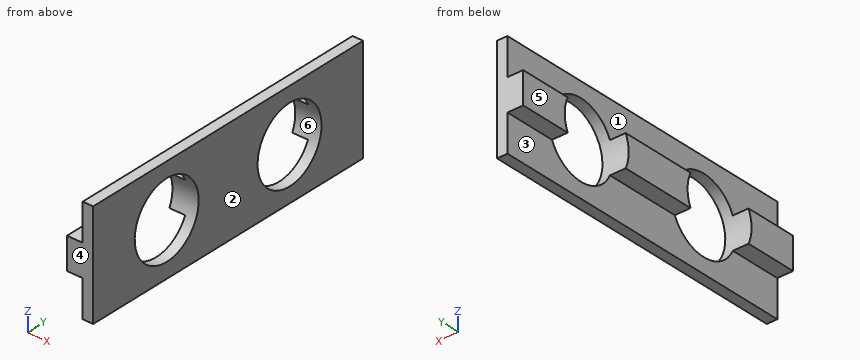
from build123d import *

# Parameters (mm, degrees)
BOSS_EXTRUDE1_DEPTH = 30
SKETCH2_R           = 3.556
CUT_EXTRUDE1_DEPTH  = 30


with BuildPart() as part:
    # Sketch1 → Boss-Extrude1 (new body)
    with BuildSketch(Plane(origin=(0, 0, 0), x_dir=(1, 0, 0), z_dir=(0, 1, 0))):
        Polygon((-1.62605042, 3), (-1.62605042, 6.5), (-0.62605042, 6.5), (-0.62605042, -3.5), (-1.62605042, -3.5), (-1.62605042, 0), (-3.12605042, 0), (-3.12605042, 3), align=None)
    extrude(amount=BOSS_EXTRUDE1_DEPTH)

    # Sketch2 → Cut-Extrude1 (cut)
    with BuildSketch(Plane.ZY.offset(3.12605042)):
        with Locations((-1.5, 21.829992104)):
            Circle(SKETCH2_R)
        with Locations((-1.5, 8.170007896)):
            Circle(SKETCH2_R)
    extrude(amount=-CUT_EXTRUDE1_DEPTH, mode=Mode.SUBTRACT)


solid = part.part
Could you check a few things on this model? Use its own coordinates, in mm. Face numbers are marked on the shaded views. A direction names the side the tool comes from. Coordinates: 2 decimals unless noted, no trailing zeros. Write each loop counter-clockwise with the first axis right and the second up, starting at its lowest first coordinate (ties: lowest second). Pieces come first, ordered by that corner, then holes. Notation, with made-up numbers: (60.5, -23.5) - (117.5, -23.5) arc R33 cw to (117.5, 11.5) - close; hole circle Ø4 at (37, 68). An arc over 180 degrees is marked (long way). Put each result on its own line as item: value. Start each with the question number.
Q1. I want a section at B-B on y = 20. Write out the boundary of the cut face in (x, z).
Q2. Thinking about a two-plate mould opening in Y: for the marked faces 4, 5 and 6, which applies, pulls with the +Y half, pulls with the -Y half, needs draft (parallel to the pull), parting line crosses it, or undercut?
Q3. Please list where these lines run through material, in increasing order: L1, parallel to Y at x = -2.5, z = -1.5; L2, parallel to Y at x = -1.45, z = 1.5; L3, parallel to Z at x = -1.4, y = 8.
Q4. Which directions (+Z, -Z, +X, -X, +Y, -Y) give clear straight access to the entire face, cutting with the end or side of a thin tool? Please do the marked faces 1, 2 and 3.
Q5. I want a section at C-C on z = 1.75. Write out the boundary of the cut face in (x, y).
Q6. I'm going to push flat-ended pins straight in: P1, Ø6, axis at y = 22, z = -0.5, coming from the -X side; P2, Ø5.5, axis at y = 21.83, z = -1.5, coming from the +X side. Where does each tip first touch, or does it pass through?
Q7. I want a section at A-A on x = -2.15. Write out the boundary of the cut face in (y, z).
Checks:
1. outline: (-1.63, -6.5) - (-0.63, -6.5) - (-0.63, -4.55) - (-1.63, -4.55) - close; (-1.63, 1.55) - (-0.63, 1.55) - (-0.63, 3.5) - (-1.63, 3.5) - close
2. face 4: pulls with the -Y half
2. face 5: needs draft
2. face 6: undercut
3. L1: 0 to 4.61, 11.73 to 18.27, 25.39 to 30
3. L2: 0 to 6.26, 10.08 to 19.92, 23.74 to 30
3. L3: -6.5 to -5.05, 2.05 to 3.5
4. face 1: +Z, -X, +Y, -Y
4. face 2: +Z, -Z, +X, +Y, -Y
4. face 3: -Z, -X, +Y, -Y
5. outline: (-1.63, 0) - (-0.63, 0) - (-0.63, 6.73) - (-1.63, 6.73) - close; (-1.63, 9.61) - (-0.63, 9.61) - (-0.63, 20.39) - (-1.63, 20.39) - close; (-1.63, 23.27) - (-0.63, 23.27) - (-0.63, 30) - (-1.63, 30) - close
6. P1: x = -1.63
6. P2: through
7. outline: (0, -3) - (4.95, -3) arc R3.56 cw to (4.95, 0) - (0, 0) - close; (11.39, -3) - (18.61, -3) arc R3.56 cw to (18.61, 0) - (11.39, 0) arc R3.56 cw to start; (25.05, -3) - (30, -3) - (30, 0) - (25.05, 0) arc R3.56 cw to start
